from build123d import *

# Parameters (mm, degrees)
FRONTSKETCH_W       = 17
FRONTSKETCH_H       = 61
BOSS_EXTRUDE1_DEPTH = 40
FILLET1_R           = 5


with BuildPart() as part:
    # FrontSketch → Boss-Extrude1 (new body)
    with BuildSketch(Plane.XY):
        Rectangle(FRONTSKETCH_W, FRONTSKETCH_H)
    extrude(amount=BOSS_EXTRUDE1_DEPTH)

    # Fillet1
    fillet1_edges = [part.edges().sort_by_distance(p)[0] for p in [
        (8.5, 0, 40),
        (0, 30.5, 40),
        (-8.5, 0, 40),
        (0, 30.5, 0),
        (8.5, 0, 0),
        (0, -30.5, 0),
        (-8.5, 0, 0),
        (-8.5, 30.5, 20),
        (8.5, 30.5, 20),
        (8.5, -30.5, 20),
        (-8.5, -30.5, 20),
        (0, -30.5, 40),
    ]]
    fillet(fillet1_edges, radius=FILLET1_R)


solid = part.part
Geometry check sheet. Reference: the model listing, model coordinates, mm. Round coordinates to 2 decimals unless told otherwise and drop trailing zeros. Loops run counter-clockwise (first coordinate to the right, second up) from the corner with the lowest first, then second, coordinate; pieces in that order, holes last.
Item 1: Cross-section at B-B on z = 11. Record the boundary of the cut face in (x, y), then the cut area to 3 significant figures.
Item 2: Gauge pin test, flat ends, axial feed: pin 1 (3 mm diameter, centred on x = 5.5, z = 12.5, fed in from -Y); pin 2 (3 mm diameter, centred on x = 5.5, z = 19, fed in from +Y). Record the tip position at first contact, or that the pin passes through.
Item 3: Cross-section at A-A on y = 7. Record the boundary of the cut face in (x, z), then the cut area to 3 significant figures.
Item 4: Thickness scan on line 1 (Z direction, x = -3.75, y = 15.5); line 2 (Z direction, x = 5.5, y = -8); line 3 (X direction, y = -5.5, z = 38). Record the ranges inside material, lowest first.
Answer sheet:
1. outline: (-8.5, -25.5) arc R5 ccw to (-3.5, -30.5) - (3.5, -30.5) arc R5 ccw to (8.5, -25.5) - (8.5, 25.5) arc R5 ccw to (3.5, 30.5) - (-3.5, 30.5) arc R5 ccw to (-8.5, 25.5) - close
1. area: 1,020 mm2
2. pin 1: stops at y = -30.47
2. pin 2: stops at y = 30.47
3. outline: (-8.5, 5) arc R5 ccw to (-3.5, 0) - (3.5, 0) arc R5 ccw to (8.5, 5) - (8.5, 35) arc R5 ccw to (3.5, 40) - (-3.5, 40) arc R5 ccw to (-8.5, 35) - close
3. area: 659 mm2
4. line 1: z = 0.01 to 39.99
4. line 2: z = 0.42 to 39.58
4. line 3: x = -7.5 to 7.5
